Geometry: final body of the model. Coordinates: model frame, mm. Give positions to 0.01 mm unless a question says otherwise; leave off trailing zeros. Write each loop counter-clockwise with the first axis right and the second up, starting at its lowest first coordinate (ties: lowest second). Pieces come first, ordered by that corner, then holes.
from build123d import *

# Parameters (mm, degrees)
SKETCH1_W           = 6.35
SKETCH1_H           = 40
BOSS_EXTRUDE1_DEPTH = 6.35
SKETCH2_W           = 3.175
SKETCH2_H           = 6.604
CUT_EXTRUDE1_DEPTH  = 622.232333753


with BuildPart() as part:
    # Sketch1 → Boss-Extrude1 (new body)
    with BuildSketch(Plane.XY):
        Polygon((0, 0), (420, 0), (420, 457.7), (413.65, 457.7), (407.3, 457.7), (12.7, 457.7), (6.35, 457.7), (0, 457.7), align=None)
        with Locations((9.525, 385)):
            Rectangle(SKETCH1_W, SKETCH1_H, mode=Mode.SUBTRACT)
        with Locations((410.475, 385)):
            Rectangle(SKETCH1_W, SKETCH1_H, mode=Mode.SUBTRACT)
        with Locations((9.525, 230)):
            Rectangle(SKETCH1_W, SKETCH1_H, mode=Mode.SUBTRACT)
        with Locations((410.475, 230)):
            Rectangle(SKETCH1_W, SKETCH1_H, mode=Mode.SUBTRACT)
        with Locations((410.475, 75)):
            Rectangle(SKETCH1_W, SKETCH1_H, mode=Mode.SUBTRACT)
        with Locations((9.525, 75)):
            Rectangle(SKETCH1_W, SKETCH1_H, mode=Mode.SUBTRACT)
    extrude(amount=BOSS_EXTRUDE1_DEPTH)

    # Sketch2 → Cut-Extrude1 (cut, through all)
    with BuildSketch(Plane(origin=(420, 0, 0), x_dir=(0, 0, -1), z_dir=(1, 0, 0))):
        with Locations((-4.7625, 448.302)):
            Rectangle(SKETCH2_W, SKETCH2_H)
    extrude(amount=-CUT_EXTRUDE1_DEPTH, mode=Mode.SUBTRACT)


solid = part.part
Q1. Pin query (flat end, axial travel): P1, Ø2, axis at x = 128.5, y = 450, coming from the +Z side (3 decimals). Return the tip coordinate at first contact, or that it passes through.
Filled sheet:
P1: stops at z = 3.175
Q2. Section B-B on y = 61.5. Output: boundary loops of the cut face in (x, z).
Filled sheet:
outline: (0, 0) - (6.35, 0) - (6.35, 6.35) - (0, 6.35) - close; (12.7, 0) - (407.3, 0) - (407.3, 6.35) - (12.7, 6.35) - close; (413.65, 0) - (420, 0) - (420, 6.35) - (413.65, 6.35) - close
Q3. Section A-A on z = 4.75. Count the separate pieces of the cut face and the enclosed holes in it, plus the area to 3 significant figures.
Filled sheet:
separate pieces: 2
enclosed holes: 6
area: 188,000 mm2
Q4. Ray query, line 1 along X through (y, z) = (79, 1); line 2 along Y through (x, z) = (203, 5.25). Return the intervals inside material, ascending.
Filled sheet:
line 1: x = 0 to 6.35, 12.7 to 407.3, 413.65 to 420
line 2: y = 0 to 445, 451.6 to 457.7
